Source: CAD feature listing. Evaluate the final solid. Frame: model axes, mm. Face numbers are marked on the shaded views. A direction names the side the tool comes from. Give positions to 0.01 mm unless a question says otherwise; leave off trailing zeros. Order: outer loops, then holes, each group sorted by start corner. A loop starts at its lowest first (then second) coordinate and runs counter-clockwise, first axis right, second up. Notation, with made-up numbers: (34.5, 4) -> (79.5, 4) arc R7 cw to (79.5, 14) -> close; hole circle Ø6 at (47, 72.5). An arc over 180 degrees is marked (long way). Answer in a Markdown table with one row per item.
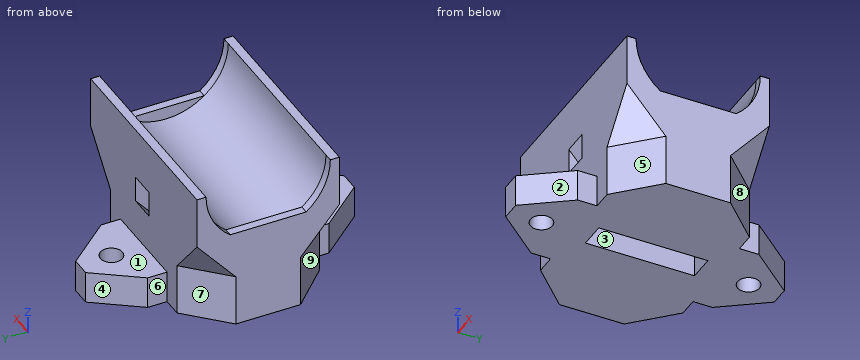
```python
from build123d import *
from OCP.BRepFilletAPI import BRepFilletAPI_MakeChamfer
from build123d.topology import SkipClean

# Parameters (mm, degrees)
BOSS_EXTRU_1_DEPTH           = 15
ENL_V_START                  = -1.3
ESQUISSE2_R                  = 9.6
ENL_V_MAT_EXTRU_1_DEPTH      = 29.4
ENL_V_MAT_EXTRU_2_DEPTH      = 36.895542898805694
ENL_V_MAT_EXTRU_2_DEPTH_BACK = 36.895542898805694
BOSS_EXTRU_2_DEPTH           = 3
ESQUISSE6_R                  = 1.7
ENL_V_MAT_EXTRU_3_DEPTH      = 30.000000000000014
CHANFREIN1_SIZE              = 5
CHANFREIN1_SIZE2             = 7
CHANFREIN2_SIZE              = 7
CHANFREIN2_SIZE2             = 6
CHANFREIN3_START             = 12.698865856
CHANFREIN3_OUTLINE_W         = 11
CHANFREIN3_OUTLINE_H         = 12.000000000000002
CHANFREIN3_DEPTH             = 4.301134144
CHANFREIN4_START             = 12.698865856
CHANFREIN4_OUTLINE_W         = 11
CHANFREIN4_OUTLINE_H         = 12.000000000000002
CHANFREIN4_DEPTH             = 4.301134144
CHANFREIN5_START             = -17
CHANFREIN5_OUTLINE_W         = 11
CHANFREIN5_OUTLINE_H         = 12.000000000000002
CHANFREIN5_DEPTH             = 4.301134144
CHANFREIN6_START             = -17
CHANFREIN6_OUTLINE_W         = 11
CHANFREIN6_OUTLINE_H         = 12.000000000000002
CHANFREIN6_DEPTH             = 4.301134144
ENL_V_START_2                = -13.5
ENL_V_MAT_EXTRU_4_DEPTH      = 4
ESQUISSE10_R                 = 1.6999999999999995
ESQUISSE10_R_2               = 1.7000000000000002
ESQUISSE10_W                 = 4
ESQUISSE10_H                 = 16.857142857142858
BOSS_EXTRU_3_DEPTH           = 8
ESQUISSE12_W                 = 14
ESQUISSE12_H                 = 9.999999999999995
ESQUISSE12_W_2               = 14.000000000000002
ESQUISSE12_H_2               = 9.999999999999996
ENL_V_MAT_EXTRU_6_DEPTH      = 6


with BuildPart() as part:
    # Esquisse1 → Boss.-Extru.1 (new body)
    with BuildSketch(Plane.XY):
        Polygon((-16.000000000000007, 11.000000000000002), (15.999999999999993, 11.000000000000002), (15.999999999999996, -11), (-16, -11), align=None)
    extrude(amount=BOSS_EXTRU_1_DEPTH)

    # Esquisse2 → Enlèv. mat.-Extru.1 (cut)
    with BuildSketch(Plane(origin=(15.999999999999996, 2.52e-15, 0), x_dir=(0, 0, -1), z_dir=(1, 1.6e-16, 0)).offset(ENL_V_START)):
        with Locations((-15, -1.73e-15)):
            Circle(ESQUISSE2_R)
    extrude(amount=-ENL_V_MAT_EXTRU_1_DEPTH, mode=Mode.SUBTRACT)

    # Esquisse4 → Enlèv. mat.-Extru.2 (cut, two sides: drawn at the far end of the back side and taken through both)
    with SkipClean():  # the faces are left unmerged after this step: merging them gives an invalid solid
        with BuildSketch(Plane(origin=(-14.700000000000001, -2.32e-15, 0), x_dir=(0, 0, -1), z_dir=(1, 1.6e-16, 0)).offset(-ENL_V_MAT_EXTRU_2_DEPTH_BACK)):
            with BuildLine():
                Line((-7.3999999999999995, -5.865151319446073), (-7.3999999999999995, 5.865151319446073))
                ThreePointArc((-7.3999999999999995, 5.865151319446073), (-10.76593886833709, 8.615841591704243), (-15.000000000000032, 9.599999999999998))
                Line((-15.000000000000032, 9.599999999999998), (-15, -9.600000000000001))
                ThreePointArc((-15, -9.600000000000001), (-10.765938868337066, -8.615841591704251), (-7.3999999999999995, -5.865151319446073))
            make_face()
        extrude(amount=ENL_V_MAT_EXTRU_2_DEPTH + ENL_V_MAT_EXTRU_2_DEPTH_BACK, mode=Mode.SUBTRACT)

    # Esquisse5 → Boss.-Extru.2 (add)
    with BuildSketch(Plane(origin=(0, 0, 0), x_dir=(-1, 0, 0), z_dir=(0, 0, -1))):
        Polygon((7.000000000000008, -11), (-6.999999999999992, -11.000000000000002), (-6.999999999999991, -20.999999999999993), (7.000000000000009, -20.999999999999996), align=None)
        Polygon((7.000000000000006, 11.000000000000002), (-6.999999999999994, 11), (-6.999999999999992, 20.999999999999996), (7.000000000000008, 20.999999999999996), align=None)
    extrude(amount=-BOSS_EXTRU_2_DEPTH)

    # Esquisse6 → Enlèv. mat.-Extru.3 (cut, through all)
    with BuildSketch(Plane.XY.offset(3)):
        with Locations((0, -15.999999999999996)):
            Circle(ESQUISSE6_R)
        with Locations((8.7e-16, 15.999999999999996)):
            Circle(ESQUISSE6_R)
    extrude(amount=-ENL_V_MAT_EXTRU_3_DEPTH, mode=Mode.SUBTRACT)

    # Chanfrein1: one chamfer whose edges measure the first distance from different faces: ONE call of the kernel's chamfer builder (chamfer() names one face for all edges)
    chanfrein1_edges_1 = [part.edges().sort_by_distance(p)[0] for p in [
        (6.999999999999991, -20.999999999999993, 1.5),
    ]]
    chanfrein1_side_1 = [part.faces().sort_by_distance(p)[0] for p in [
        (-9.13e-15, -20.999999999999993, 1.5),
    ]]
    chanfrein1_edges_2 = [part.edges().sort_by_distance(p)[0] for p in [
        (-7.000000000000008, 20.999999999999996, 1.5),
    ]]
    chanfrein1_side_2 = [part.faces().sort_by_distance(p)[0] for p in [
        (-8.24e-15, 20.999999999999996, 1.5),
    ]]
    chanfrein1 = BRepFilletAPI_MakeChamfer(part.part.solid().wrapped)
    for e in chanfrein1_edges_1:
        chanfrein1.Add(CHANFREIN1_SIZE, CHANFREIN1_SIZE2, e.wrapped, chanfrein1_side_1[0].wrapped)  # the first distance lies on this face
    for e in chanfrein1_edges_2:
        chanfrein1.Add(CHANFREIN1_SIZE, CHANFREIN1_SIZE2, e.wrapped, chanfrein1_side_2[0].wrapped)  # the first distance lies on this face
    add(Compound.cast(chanfrein1.Shape()), mode=Mode.REPLACE)

    # Chanfrein2: one chamfer whose edges measure the first distance from different faces: ONE call of the kernel's chamfer builder (chamfer() names one face for all edges)
    chanfrein2_edges_1 = [part.edges().sort_by_distance(p)[0] for p in [
        (6.999999999999992, 20.999999999999996, 1.5),
    ]]
    chanfrein2_side_1 = [part.faces().sort_by_distance(p)[0] for p in [
        (6.999999999999993, 15.999999999999998, 1.5),
    ]]
    chanfrein2_edges_2 = [part.edges().sort_by_distance(p)[0] for p in [
        (-7.000000000000009, -20.999999999999996, 1.5),
    ]]
    chanfrein2_side_2 = [part.faces().sort_by_distance(p)[0] for p in [
        (-7.000000000000009, -15.999999999999998, 1.5),
    ]]
    chanfrein2 = BRepFilletAPI_MakeChamfer(part.part.solid().wrapped)
    for e in chanfrein2_edges_1:
        chanfrein2.Add(CHANFREIN2_SIZE, CHANFREIN2_SIZE2, e.wrapped, chanfrein2_side_1[0].wrapped)  # the first distance lies on this face
    for e in chanfrein2_edges_2:
        chanfrein2.Add(CHANFREIN2_SIZE, CHANFREIN2_SIZE2, e.wrapped, chanfrein2_side_2[0].wrapped)  # the first distance lies on this face
    add(Compound.cast(chanfrein2.Shape()), mode=Mode.REPLACE)

    # Chanfrein3: read off the stored shape, not the designer's step
    # Chanfrein3 outline → Chanfrein3 (cut)
    with BuildSketch(Plane(origin=(0, 0, 0), x_dir=(0.7964473354898962, 0.4591284639882932, 0.39353868341853704), z_dir=(0.6047078979069521, -0.6047078979069521, -0.5183210553488161)).offset(CHANFREIN3_START)):
        with Locations((6.5, 8)):
            Rectangle(CHANFREIN3_OUTLINE_W, CHANFREIN3_OUTLINE_H)
    extrude(amount=CHANFREIN3_DEPTH, mode=Mode.SUBTRACT)

    # Chanfrein4: read off the stored shape, not the designer's step
    # Chanfrein4 outline → Chanfrein4 (cut)
    with BuildSketch(Plane(origin=(0, 0, 0), x_dir=(0.7964473354898962, -0.45912846398829327, 0.39353868341853704), z_dir=(0.6047078979069521, 0.6047078979069522, -0.5183210553488161)).offset(CHANFREIN4_START)):
        with Locations((6.5, -8)):
            Rectangle(CHANFREIN4_OUTLINE_W, CHANFREIN4_OUTLINE_H)
    extrude(amount=CHANFREIN4_DEPTH, mode=Mode.SUBTRACT)

    # Chanfrein5: read off the stored shape, not the designer's step
    # Chanfrein5 outline → Chanfrein5 (cut)
    with BuildSketch(Plane(origin=(0, 0, 0), x_dir=(0.7964473354898962, 0.45912846398829327, -0.39353868341853704), z_dir=(0.6047078979069521, -0.6047078979069522, 0.5183210553488161)).offset(CHANFREIN5_START)):
        with Locations((-6.5, 8)):
            Rectangle(CHANFREIN5_OUTLINE_W, CHANFREIN5_OUTLINE_H)
    extrude(amount=CHANFREIN5_DEPTH, mode=Mode.SUBTRACT)

    # Chanfrein6: read off the stored shape, not the designer's step
    # Chanfrein6 outline → Chanfrein6 (cut)
    with BuildSketch(Plane(origin=(0, 0, 0), x_dir=(0.796447335489896, -0.45912846398829327, -0.39353868341853715), z_dir=(0.6047078979069522, 0.6047078979069521, 0.5183210553488161)).offset(CHANFREIN6_START)):
        with Locations((-6.5, -8)):
            Rectangle(CHANFREIN6_OUTLINE_W, CHANFREIN6_OUTLINE_H)
    extrude(amount=CHANFREIN6_DEPTH, mode=Mode.SUBTRACT)

    # Esquisse7 → Enlèv. mat.-Extru.4 (cut)
    with BuildSketch(Plane(origin=(15.999999999999996, 2.52e-15, 0), x_dir=(0, 0, -1), z_dir=(1, 1.6e-16, 0)).offset(ENL_V_START_2)):
        Polygon((-3, -7.571428571428581), (-3, 7.571428571428564), (-7.000000000000009, 11), (-3.000000000000009, 11), (-4.5e-16, 8.428571428571422), (1.83e-15, -8.428571428571436), (-2.999999999999989, -11.000000000000002), (-6.9999999999999885, -11.000000000000002), align=None)
    extrude(amount=-ENL_V_MAT_EXTRU_4_DEPTH, mode=Mode.SUBTRACT)

    # Esquisse10 → Boss.-Extru.3 (add)
    with BuildSketch(Plane(origin=(0, 0, 0), x_dir=(-1, 0, 0), z_dir=(0, 0, -1))):
        Polygon((-9.999999999999998, -11.000000000000004), (-15.999999999999996, -5.000000000000007), (-15.999999999999993, 4.999999999999996), (-9.999999999999995, 11), (-6.999999999999994, 11), (-6.999999999999993, 13.999999999999977), (-0.9999999999999818, 20.999999999999996), (1.999999999999995, 20.999999999999996), (7.000000000000008, 13.999999999999968), (7.000000000000006, 11.000000000000002), (10.000000000000009, 11.000000000000004), (16.000000000000004, 5.000000000000002), (16.000000000000007, -4.999999999999992), (9.999999999999993, -11), (7.000000000000008, -11), (7.000000000000008, -13.999999999999963), (0.99999999999999, -20.999999999999996), (-1.9999999999999645, -20.999999999999993), (-6.999999999999992, -13.999999999999954), (-6.999999999999992, -11), align=None)
        with Locations(Location((-8.7e-16, 15.999999999999996, 0), (0, 0, 180))):
            Circle(ESQUISSE10_R, mode=Mode.SUBTRACT)
        with Locations(Location((0, -15.999999999999996, 0), (0, 0, 180))):
            Circle(ESQUISSE10_R_2, mode=Mode.SUBTRACT)
        with Locations((-0.499999999999997, -7.11e-15)):
            Rectangle(ESQUISSE10_W, ESQUISSE10_H, mode=Mode.SUBTRACT)
    extrude(amount=BOSS_EXTRU_3_DEPTH)

    # Esquisse12 → Enlèv. mat.-Extru.6 (cut)
    with BuildSketch(Plane.XY.offset(3)):
        with Locations((-5.77e-15, 16)):
            Rectangle(ESQUISSE12_W, ESQUISSE12_H)
        with Locations((-7.11e-15, -15.999999999999998)):
            Rectangle(ESQUISSE12_W_2, ESQUISSE12_H_2)
    extrude(amount=-ENL_V_MAT_EXTRU_6_DEPTH, mode=Mode.SUBTRACT)


solid = part.part
```
(1) First-contact query: pin 1 Ø1 at (x, y) = (-5, -12.5) entering from +Z; pin 2 Ø5 at (x, z) = (10.5, 0) entering from +Y; pin 3 Ø1.5 at (y, z) = (13, -5) entering from -X. Flat tips, straight axial feed; report the tip coordinate or a pass-through.
A:
| item | result |
|---|---|
| pin 1 | stops at z = -3 |
| pin 2 | stops at y = 11 |
| pin 3 | stops at x = -7 |
(2) Section query D-D (z = 1.5). Return the cut outline in (x, y).
A:
| item | result |
|---|---|
| outline | (-16, -6.29) -> (-11.29, -11) -> (11.29, -11) -> (16, -6.29) -> (16, 6.29) -> (11.29, 11) -> (-11.29, 11) -> (-16, 6.29) -> close; hole (-1.5, -9.71) -> (2.5, -9.71) -> (2.5, 9.71) -> (-1.5, 9.71) -> close |
(3) Ray query, probe 1 along Y at (x, z) = (0, -5.05); probe 2 along Y at (x, z) = (-13, 3.75); probe 3 along X at (y, z) = (16, -5.45). Return the intervals inside material, ascending.
A:
| item | result |
|---|---|
| probe 1 | y = -21 to -17.7, -14.3 to -8.43, 8.43 to 14.3, 17.7 to 21 |
| probe 2 | y = -11 to 11 |
| probe 3 | x = -5.57 to -1.7, 1.7 to 5.29 |
(4) Section query C-C (y = -16). Return the cut outline in (x, z).
A:
| item | result |
|---|---|
| outline | (-5.29, -8) -> (-1.7, -8) -> (-1.7, -3) -> (-5.29, -3) -> close; (1.7, -8) -> (5.57, -8) -> (5.57, -3) -> (1.7, -3) -> close |
(5) Access query for the marked faces 5, 6, 7, 8 and 9. Directions: +Z, -Z, +X, -X, +Y, -Y. A direction counts if a zero-diameter tool reaches every point of the face in a straight line with its end or side. Return the directions, or none.
A:
| item | result |
|---|---|
| face 5 | -Z, +X, -Y |
| face 6 | +Z, -Z, -X, +Y |
| face 7 | -Z, -X, +Y |
| face 8 | -Z, +X, +Y |
| face 9 | -Z, -X, -Y |
(6) Section query B-B (z = -4.75). Return the cut outline in (x, y).
A:
| item | result |
|---|---|
| outline | (-16, -5) -> (-10, -11) -> (-7, -11) -> (-7, -14) -> (-1, -21) -> (2, -21) -> (7, -14) -> (7, -11) -> (10, -11) -> (16, -5) -> (16, 5) -> (10, 11) -> (7, 11) -> (7, 14) -> (1, 21) -> (-2, 21) -> (-7, 14) -> (-7, 11) -> (-10, 11) -> (-16, 5) -> close; hole circle Ø3.4 at (0, -16); hole circle Ø3.4 at (0, 16); hole (-1.5, -8.43) -> (2.5, -8.43) -> (2.5, 8.43) -> (-1.5, 8.43) -> close |
(7) Section query A-A (x = 0). Return the cut outline in (y, z), plus the area to 3 significant figures.
A:
| item | result |
|---|---|
| outline | (-21, -8) -> (-17.7, -8) -> (-17.7, -3) -> (-21, -3) -> close; (-14.3, -8) -> (-8.43, -8) -> (-8.43, 0) -> (-11, 3) -> (-11, -3) -> (-14.3, -3) -> close; (-11, 7) -> (-7.57, 3) -> (7.57, 3) -> (11, 7) -> (11, 15) -> (9.6, 15) arc R9.6 cw to (-9.6, 15) -> (-11, 15) -> close; (8.43, -8) -> (14.3, -8) -> (14.3, -3) -> (11, -3) -> (11, 3) -> (8.43, 0) -> close; (17.7, -8) -> (21, -8) -> (21, -3) -> (17.7, -3) -> close |
| area | 220 mm^2 |
(8) Pull-direction query (X, two-part tool) for the marked faces 1, 2, 3 and 4; classes: +X half, -X half, draft (parallel to the pull), parting line (faces both ways), or undercut.
A:
| item | result |
|---|---|
| face 1 | draft |
| face 2 | +X half |
| face 3 | undercut |
| face 4 | -X half |
